Input: part model. Units: mm. Frame: model coordinates. Give positions to 0.01 mm unless a question says otherwise; leave off trailing zeros. Write each loop counter-clockwise with the first axis right and the second up, starting at its lowest first coordinate (ties: lowest second). Pieces come first, ordered by that corner, then holes. Notation, with made-up numbers: (75.25, -20) -> (106.25, -20) arc R26 cw to (106.25, 8) -> close; hole circle Ø11 at (28, 29.5). An arc over 180 degrees is marked (long way). Return JSON: item names as keys, results as strings. Group by question number.
Item 1: Section A-A, the plane z = 2.8. Return loops of the section in (x, y), then the cut area to 3 significant figures.
Item 2: Pin query (flat end, axial travel): P1, Ø2, axis at x = 2.5, z = 3, coming from the +Y side; P2, Ø1, axis at x = 10, z = 2, coming from the -Y side. Return the tip coordinate at first contact, or that it passes through.
Item 3: Mould query, pull axis Y, two halves, no side actions, for faces 1 (the face through (-12.253, 75.024, 1.972)), 2 (the face through (-0.6, 59.62, 1.97)), 3 (the face through (0, 41, 4)). Classes: released by +Y, released by -Y, zero draft, split by the parting line, or undercut.
Item 4: Section C-C, the plane y = 74. Return loops of the section in (x, z), then the cut area to 3 significant figures.
Item 5: Line query: line 1 (Y direction, x = 0.05, z = 1.65); line 2 (Y direction, x = -2.5, z = 0.3); line 3 (X direction, y = 63, z = 2.8). Output: solid intervals per line, ascending. Write a range as [from, to].
Item 6: Section B-B, the plane x = -7.5. Return loops of the section in (y, z), then the cut area to 3 significant figures.
from build123d import *

# Parameters (mm, degrees)
SKETCH_1_R      = 3
EXTRUDE_1_DEPTH = 4


with BuildPart() as part:
    # Эскиз1 → Бобышка-Вытянуть1 (new body)
    with BuildSketch(Plane.XY):
        with BuildLine():
            Line((-17.5, 0), (17.5, 0))
            Line((17.5, 0), (17.5, 62.55))
            ThreePointArc((17.5, 62.55), (12.389013332, 74.889013332), (0.05, 80))
            Line((0.05, 80), (-0.05, 80))
            ThreePointArc((-0.05, 80), (-12.389013332, 74.889013332), (-17.5, 62.55))
            Line((-17.5, 62.55), (-17.5, 0))
        make_face()
        with Locations((0.05, 62.55)):
            Circle(SKETCH_1_R, mode=Mode.SUBTRACT)
    extrude(amount=EXTRUDE_1_DEPTH)


solid = part.part
Answer below:
{
 "1": {"outline": "(-17.5, 0) -> (17.5, 0) -> (17.5, 62.55) arc R17.45 ccw to (0.05, 80) -> (-0.05, 80) arc R17.45 ccw to (-17.5, 62.55) -> close; hole circle Ø6 at (0.05, 62.55)", "area": "2,640 mm2"},
 "2": {"P1": "stops at y = 79.94", "P2": "stops at y = 0"},
 "3": {"face 1": "released by +Y", "face 2": "undercut", "face 3": "zero draft"},
 "4": {"outline": "(-13.22, 0) -> (13.22, 0) -> (13.22, 4) -> (-13.22, 4) -> close", "area": "106 mm2"},
 "5": {"line 1": "y = [0, 59.55], [65.55, 80]", "line 2": "y = [0, 60.97], [64.13, 79.83]", "line 3": "x = [-17.49, -2.92], [3.02, 17.49]"},
 "6": {"outline": "(0, 0) -> (78.33, 0) -> (78.33, 4) -> (0, 4) -> close", "area": "313 mm2"}
}
